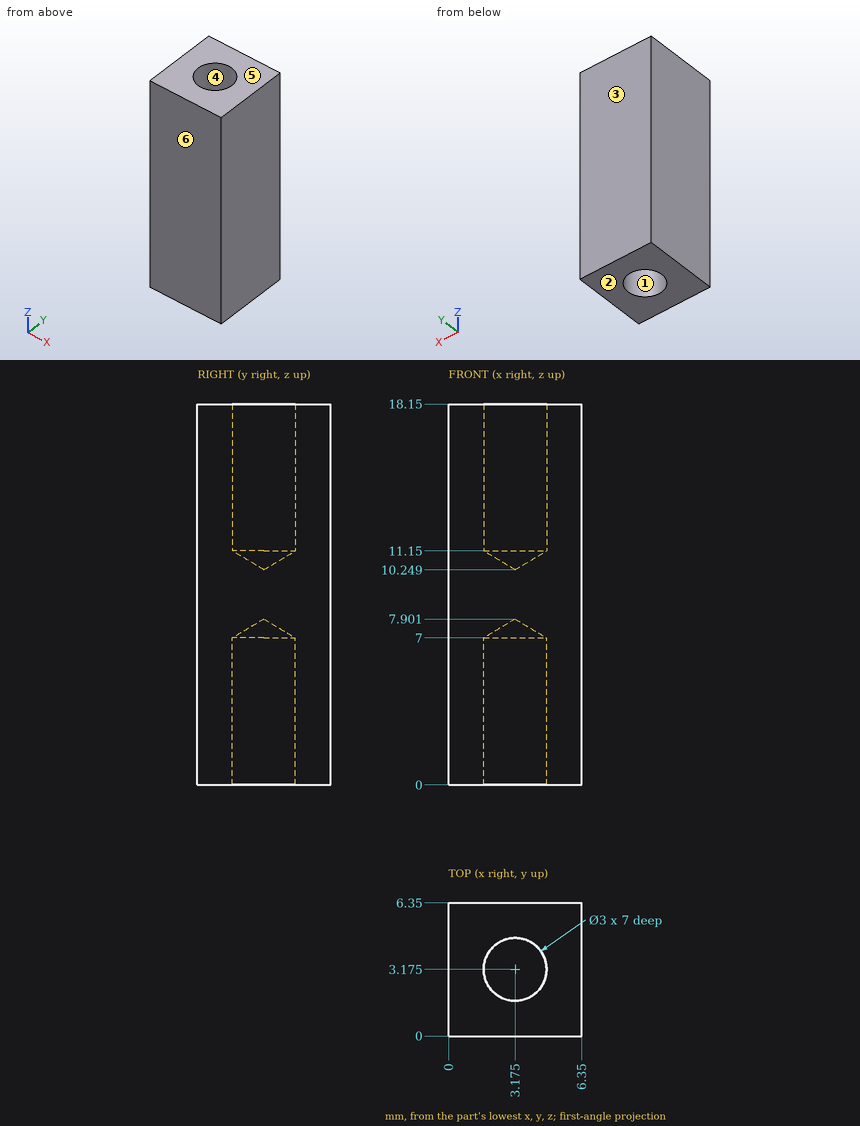
Geometry check sheet. Reference: drawing and pictorial views, mm from the part's lowest x, y, z. A direction names the side the tool comes from. Give positions to 0.01 mm unless a question says otherwise; leave off trailing zeros. Answer as a JSON object with one key per item and string values. Group by question number.
1) Mould release check, pull along Y, two halves, no side actions. Record for the marked faces 3, 4, 5 and 6: released by +Y, released by -Y, zero draft, split by the parting line, or undercut.
2) Access from +Z, -Z, +X, -X, +Y, -Y to the whole of each face (thin tool, end or side, straight path). Record for the marked faces 1 and 2.
3) Scan lines: line 1 along Y through (x, z) = (3.75, 1.25); line 2 along Y through (x, z) = (4, 2.75). Record each from-to range of solid material in increasing order. Write a range as [from, to].
4) Depth check by flat-ended pin: pin 1 Ø3 at (x, z) = (1, 6) entering from -Y; pin 2 Ø2.5 at (x, y) = (3.175, 3.175) entering from +Z. Enter the tip coordinate at first touch or a pass-through.
Result sheet:
{
 "1": {"face 3": "released by +Y", "face 4": "undercut", "face 5": "zero draft", "face 6": "released by -Y"},
 "2": {"face 1": "-Z", "face 2": "-Z, +X, -X, +Y, -Y"},
 "3": {"line 1": "y = [0, 1.79], [4.56, 6.35]", "line 2": "y = [0, 1.92], [4.43, 6.35]"},
 "4": {"pin 1": "stops at y = 0", "pin 2": "stops at z = 11"}
}
